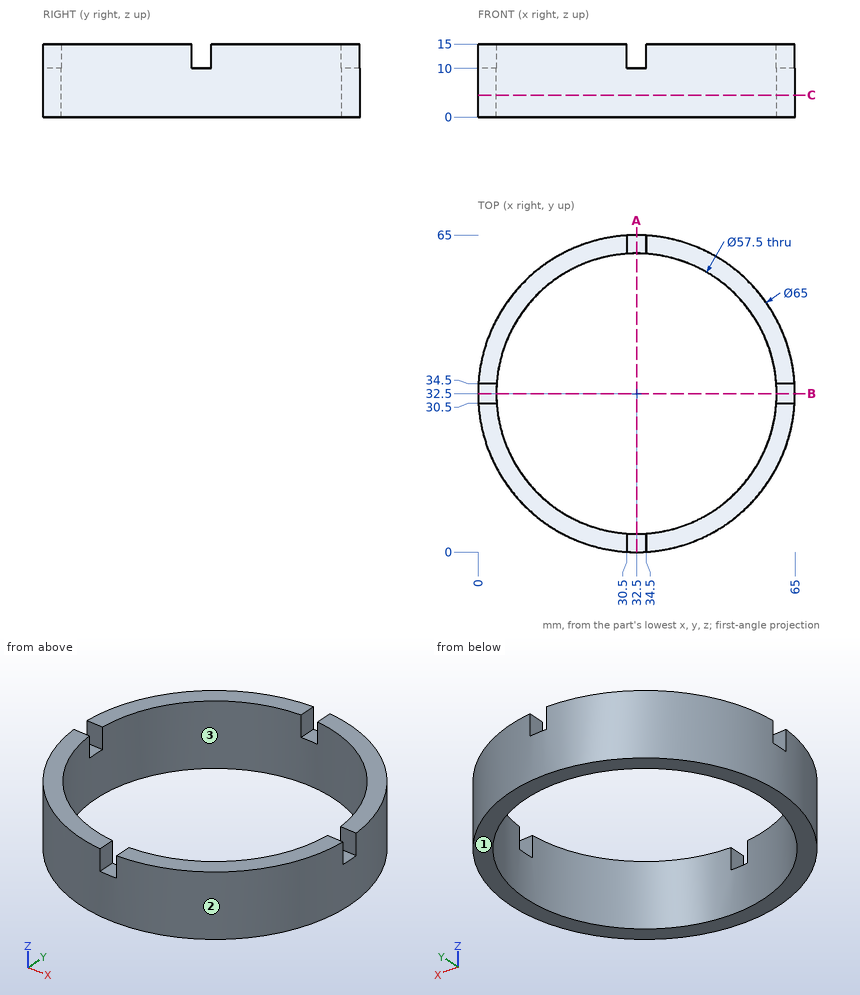
Input: dimensioned drawing with shaded views. Units: mm. Origin: part minimum x, y, z. Round coordinates to 2 decimals unless told otherwise and drop trailing zeros. Loops run counter-clockwise (first coordinate to the right, second up) from the corner with the lowest first, then second, coordinate; pieces in that order, holes last. Notation, with made-up numbers: (68, 65) -> (107, 65) arc R12 ccw to (107, 69) -> close; hole circle Ø8 at (-32.75, 14.5). An arc over 180 degrees is marked (long way). Use one line per item in the form item = value. Start each with the question number.
1) First-contact query: P1, Ø1.1, axis at x = 2.5, y = 32.5, coming from the +Z side; P2, Ø5, axis at x = 46.5, z = 3, coming from the -Y side; P3, Ø3, axis at y = 64, z = 12.5, coming from the +X side. Flat tips, straight axial feed; report the tip coordinate or a pass-through.
2) Draft query along Y for the marked faces 1, 2 and 3. Return one class per face: released by +Y, released by -Y, zero draft, split by the parting line, or undercut.
3) Line query: L1, parallel to Y at x = 32.5, z = 9.75; L2, parallel to Y at x = 19, z = 3.25. Output: solid intervals per line, ascending.
4) Section A-A on x = 32.5. Output: boundary loops of the cut face in (y, z), then the cut area to 3 significant figures.
5) Section C-C on z = 4.5. Output: boundary loops of the cut face in (x, y), then the cut area to 3 significant figures.
Response:
q1.P1 = 10
q1.P2 = 2.1
q1.P3 = 45
q2.face_1 = zero draft
q2.face_2 = split by the parting line
q2.face_3 = undercut
q3.L1 = 0 to 3.75, 61.25 to 65
q3.L2 = 2.94 to 7.12, 57.88 to 62.06
q4.outline = (0, 0) -> (3.75, 0) -> (3.75, 10) -> (0, 10) -> close; (61.25, 0) -> (65, 0) -> (65, 10) -> (61.25, 10) -> close
q4.area = 75.0 mm^2
q5.outline = circle Ø65 at (32.5, 32.5); hole circle Ø57.5 at (32.5, 32.5)
q5.area = 722 mm^2
